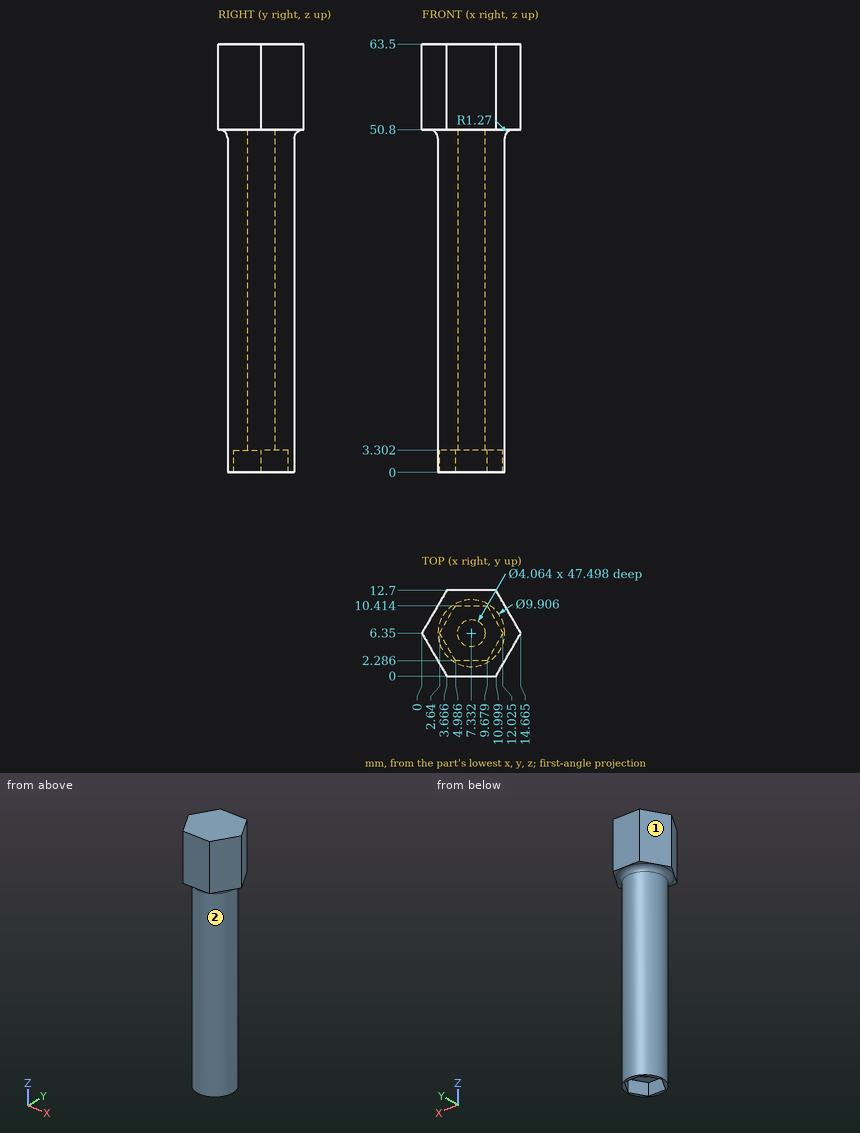
Check sheet for the drawn part. Datum: minimum x, y, z corner. Units: mm. A direction names the side the tool comes from. Give positions to 0.01 mm unless a question says otherwise; leave off trailing zeros. Answer as a JSON object with one key per item and string values.
(1) Material ranges on line 1 (X direction, y = 6.25, z = 32) (1 decimal); line 2 (Z direction, x = 4.25, y = 5.25); line 3 (X direction, y = 6, z = 23.5) (1 decimal), recorded low to high.
Report:
{"line 1": "2.4 to 5.3, 9.4 to 12.3", "line 2": "3.3 to 63.5", "line 3": "2.4 to 5.3, 9.3 to 12.3"}
(2) Depth check by flat-ended pin: pin 1 Ø2.5 at (x, z) = (8, 2) entering from +Y; pin 2 Ø4.5 at (x, y) = (7.33, 6.35) entering from -Z; pin 3 Ø2 at (y, z) = (8, 49) entering from -X. Enter the tip coordinate at first touch or a pass-through.
Report:
{"pin 1": "y = 11.3", "pin 2": "z = 3.3", "pin 3": "x = 2.42"}
(3) Tool access check on the marked faces 1 and 2. Record the directions out of +Z, -Z, +X, -X, +Y, -Y that give a thin tool (end or side, any length) a straight path to the whole face; none if there is none.
Report:
{"face 1": "+Z, -Z, -X, +Y", "face 2": "-Z"}
